CAD build for the part. Positions are in the model's coordinates, mm. A direction names the side the tool comes from. Round coordinates to 2 decimals unless told otherwise and drop trailing zeros. Write each loop counter-clockwise with the first axis right and the second up, starting at its lowest first coordinate (ties: lowest second). Pieces come first, ordered by that corner, then holes. Notation, with made-up numbers: (73, 14.5) -> (126, 14.5) arc R9 ccw to (126, 26.5) -> close; hole circle Ø10 at (55.25, 23.5). An arc over 180 degrees is marked (long way). Put each result on its own line as item: value. Start each with the question number.
1. Saw through at A-A on x = 0. List the corners of the cut face in (y, z).
2. Flat gauge pins, fed straight in: P1, Ø1.5, axis at x = 43, z = -4, coming from the +Y side; P2, Ø8, axis at x = 0, y = -3, coming from the -Z side; P3, Ø22.5, axis at x = 9, y = -5, coming from the +Z side; P4, Ø18.5, axis at x = 2, y = 0.5, coming from the -Z side. Where does each tip first touch, or does it go through?
3. Saw through at B-B on y = -18. List the corners of the cut face in (x, z).
4. Drill centre lines: line 1 (Y direction, x = 0, z = -7); line 2 (Y direction, x = 0, z = -3.05); line 3 (Z direction, x = 1, y = -9). Where is each one in solid material? Low to high. Write a range as from..to.
5. Pull direction Y, two halves, no side cores. Call faces 4 (the flat face through (16, -1, 0)), 5 (the cylindrical face through (-19.982, 0.844, -7.465)), 6 (the flat face through (33, -2.5, -5)): pulls with the +Y half, pulls with the -Y half, needs draft (parallel to the pull), parting line crosses it, or undercut.
6. Saw through at D-D on x = 19. List the corners of the cut face in (y, z) (3 decimals).
7. 3-axis set-ups, long thin cutter, end or side, ignore diameter. For faces 1 (the flat face through (-15.1, -13.4, -5)), 2 (the flat face through (9, 0, -5)), 3 (the flat face through (54.5, 0, -5)): which of +Z, -Z, +X, -X, +Y, -Y reach the whole face in a straight line?
8. Saw through at C-C on z = -3.5. List the corners of the cut face in (x, y), and give its area (3 significant figures).
from build123d import *

# Parameters (mm, degrees)
F0_R     = 8.5
F1_DEPTH = 5
F3_DEPTH = 5


with BuildPart() as f1:
    # F0 (on Top) → F1 (new body)
    with BuildSketch(Plane.XY):
        with BuildLine():
            ThreePointArc((11.224972, 2.5), (11.431036, 1.257541), (11.5, 0))
            ThreePointArc((11.5, 0), (11.431036, -1.257541), (11.224972, -2.5))
            Line((11.224972, -2.5), (54.5, -2.5))
            Line((54.5, -2.5), (54.5, 0))
            Line((54.5, 0), (54.5, 2.5))
            Line((54.5, 2.5), (11.224972, 2.5))
        make_face()
        with BuildLine():
            ThreePointArc((11.224972, -2.5), (11.431036, -1.257541), (11.5, 0))
            ThreePointArc((11.5, 0), (11.431036, 1.257541), (11.224972, 2.5))
            ThreePointArc((11.224972, 2.5), (-11.5, 0), (11.224972, -2.5))
        make_face()
        Circle(F0_R, mode=Mode.SUBTRACT)
    extrude(amount=-F1_DEPTH)

    # F2 (on face) → F3 (join)
    with BuildSketch(Plane(origin=(0, 0, -5), x_dir=(1, 0, 0), z_dir=(0, 0, -1))):
        with BuildLine():
            Line((54.5, 2.5), (22.36068, 2.5))
            ThreePointArc((22.36068, 2.5), (22.465143, 1.25194), (22.5, 0))
            ThreePointArc((22.5, 0), (22.465143, -1.25194), (22.36068, -2.5))
            Line((22.36068, -2.5), (54.5, -2.5))
            Line((54.5, -2.5), (54.5, 2.5))
        make_face()
        with BuildLine():
            ThreePointArc((19.843135, 2.5), (19.960745, 1.252458), (20, 0))
            ThreePointArc((20, 0), (19.960745, -1.252458), (19.843135, -2.5))
            Line((19.843135, -2.5), (22.36068, -2.5))
            ThreePointArc((22.36068, -2.5), (22.465143, -1.25194), (22.5, 0))
            ThreePointArc((22.5, 0), (22.465143, 1.25194), (22.36068, 2.5))
            Line((22.36068, 2.5), (19.843135, 2.5))
        make_face()
        with BuildLine():
            ThreePointArc((19.843135, -2.5), (-20, 0), (19.843135, 2.5))
            Line((19.843135, 2.5), (22.36068, 2.5))
            ThreePointArc((22.36068, 2.5), (-22.5, 0), (22.36068, -2.5))
            Line((22.36068, -2.5), (19.843135, -2.5))
        make_face()
    extrude(amount=F3_DEPTH)


solid = f1.part
Return value:
1. outline: (-22.5, -10) -> (-20, -10) -> (-20, -5) -> (-22.5, -5) -> close; (-11.5, -5) -> (-8.5, -5) -> (-8.5, 0) -> (-11.5, 0) -> close; (8.5, -5) -> (11.5, -5) -> (11.5, 0) -> (8.5, 0) -> close; (20, -10) -> (22.5, -10) -> (22.5, -5) -> (20, -5) -> close
2. P1: stops at y = 2.5
2. P2: passes through
2. P3: stops at z = 0
2. P4: stops at z = -5
3. outline: (-13.5, -10) -> (-8.72, -10) -> (-8.72, -5) -> (-13.5, -5) -> close; (8.72, -10) -> (13.5, -10) -> (13.5, -5) -> (8.72, -5) -> close
4. line 1: y = -22.5..-20, 20..22.5
4. line 2: y = -11.5..-8.5, 8.5..11.5
4. line 3: z = -5..0
5. face 4: needs draft
5. face 5: undercut
5. face 6: pulls with the -Y half
6. outline: (-12.052, -10) -> (-6.245, -10) -> (-6.245, -5) -> (-12.052, -5) -> close; (-2.5, -5) -> (2.5, -5) -> (2.5, 0) -> (-2.5, 0) -> close; (6.245, -10) -> (12.052, -10) -> (12.052, -5) -> (6.245, -5) -> close
7. face 1: +Z
7. face 2: -Z
7. face 3: +Z, -Z, +X, +Y, -Y
8. outline: (11.22, -2.5) -> (54.5, -2.5) -> (54.5, 2.5) -> (11.22, 2.5) arc R11.5 ccw (long way) to start; hole circle Ø17 at (0, 0)
8. area: 404 mm^2
